CAD build for the part. Positions are in the model's coordinates, mm. Coordinates: 2 decimals unless noted, no trailing zeros. Write each loop counter-clockwise with the first axis right and the second up, starting at its lowest first coordinate (ties: lowest second). Pieces come first, ordered by that corner, then holes. Notation, with made-up numbers: (0.25, -5) -> (15.25, -5) arc R19 ccw to (15.25, 12) -> close; hole circle Ø11 at (16.25, -7). An arc over 180 degrees is marked (long way). Answer as CSV lines item,"result".
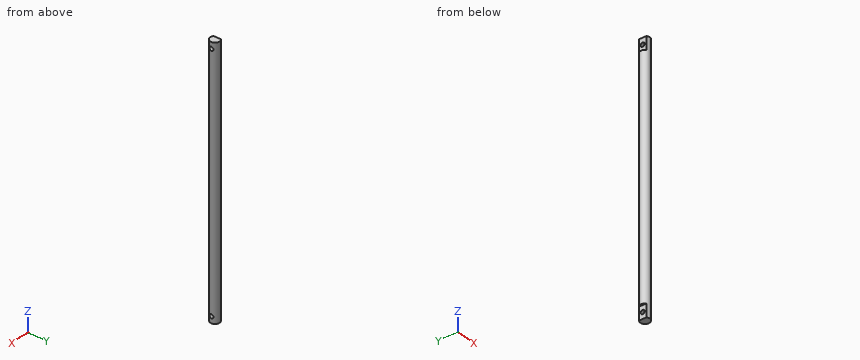
```python
from build123d import *

# Parameters (mm, degrees)
CROQUIS1_R                   = 4
SALIENTE_EXTRUIR1_DEPTH      = 223
CORTAR_EXTRUIR1_DEPTH        = 11
TALADRO_DE_MARGEN_PARA_M31_D = 3.4


with BuildPart() as part:
    # Croquis1 → Saliente-Extruir1 (new body)
    with BuildSketch(Plane.XY):
        Circle(CROQUIS1_R)
    extrude(amount=SALIENTE_EXTRUIR1_DEPTH)

    # Croquis2 → Cortar-Extruir1 (cut)
    with BuildSketch(Plane.XY.offset(223)):
        with BuildLine():
            Line((-2.5, -3.122498999), (-2.5, 3.122498999))
            ThreePointArc((-2.5, 3.122498999), (-4, 0), (-2.5, -3.122498999))
        make_face()
    cortar_extruir1 = extrude(amount=-CORTAR_EXTRUIR1_DEPTH, mode=Mode.SUBTRACT)

    # Simetría1: Cortar-Extruir1 across plane
    add(cortar_extruir1.mirror(Plane.XY.offset(111.5)), mode=Mode.SUBTRACT)

    # Taladro de margen para M31 (through all)
    with Locations(Plane(origin=(-2.5, 0, 217.5), x_dir=(0, 0, -1), z_dir=(-1, 0, 0))):
        with Locations((0, 0)):
            taladro_de_margen_para_m31 = Hole(TALADRO_DE_MARGEN_PARA_M31_D / 2)

    # Simetría3: Taladro de margen para M31 across plane
    add(taladro_de_margen_para_m31.mirror(Plane.XY.offset(111.5)), mode=Mode.SUBTRACT)


solid = part.part
```
Item 1: Saw through at C-C on z = 133. Give the cut face in (x, y).
Answer below:
outline,"circle Ø8 at (0, 0)"
Item 2: Wall check: line 1 (Z direction, x = 3.25, y = -0.75); line 2 (Z direction, x = 3.5, y = 0.5); line 3 (Y direction, x = 1.25, z = 5.5). Give the ranges that are in metal, low to high. Write a range as from..to.
Answer below:
line 1,"z = 0..3.97, 7.03..215.97, 219.03..223"
line 2,"z = 0..3.88, 7.12..215.88, 219.12..223"
line 3,"y = -3.8..-1.7, 1.7..3.8"
Item 3: Flat gauge pins, fed straight in: pin 1 (1.2 mm diameter, centred on x = -3.5, y = 1, fed in from -Z); pin 2 (1.5 mm diameter, centred on y = 2.5, z = 112.5, fed in from -X); pin 3 (3 mm diameter, centred on y = -1.5, z = 220, fed in from -X). Where does each tip first touch, or does it go through?
Answer below:
pin 1,"stops at z = 11"
pin 2,"stops at x = -3.6"
pin 3,"stops at x = -2.5"
Item 4: Saw through at A-A on y = 0. Give the cut face in (x, z), and give its area (3 significant figures).
Answer below:
outline,"(-4, 11) -> (-2.5, 11) -> (-2.5, 7.2) -> (4, 7.2) -> (4, 215.8) -> (-2.5, 215.8) -> (-2.5, 212) -> (-4, 212) -> close; (-2.5, 0) -> (4, 0) -> (4, 3.8) -> (-2.5, 3.8) -> close; (-2.5, 219.2) -> (4, 219.2) -> (4, 223) -> (-2.5, 223) -> close"
area,"1,710 mm2"
Item 5: Saw through at B-B on x = 1.5. Give the cut face in (y, z), and give its area (3 significant figures).
Answer below:
outline,"(-3.71, 0) -> (3.71, 0) -> (3.71, 223) -> (-3.71, 223) -> close; hole circle Ø3.4 at (0, 5.5); hole circle Ø3.4 at (0, 217.5)"
area,"1,640 mm2"
